Read the model definition and answer for the solid it produces. Units are mm, in the model's axes. A direction names the side the tool comes from. Give positions to 0.01 mm unless a question says otherwise; leave off trailing zeros. Loops run counter-clockwise (first coordinate to the right, second up) from the corner with the lowest first, then second, coordinate; pieces in that order, holes last. Notation, with made-up numbers: (58, 3.5) -> (98, 3.5) arc R22 ccw to (98, 13.5) -> close; hole circle Ø10 at (-26, 79). An arc over 180 degrees is marked (long way). Write each question's results on one line, items separated by ' | '. Start each with the question number.
Item 1: Determine the mould class of faces 5 (the flat face through (50, 47.625, 16)), 6 (the flat face through (101.6, 1, -4)), 7 (the flat face through (76.2, -50, 5)) for opening direction X: +X half, -X half, draft (parallel to the pull), parting line (faces both ways), or undercut.
Item 2: Which of the six approach directions +Z, -Z, +X, -X, +Y, -Y give full straight-line access (tool end or side, diameter ignored) to faces 1 (the flat face through (50, -2, 34.742)), 2 (the flat face through (25.4, -50, 5)), 3 (the flat face through (50, 7, -3.175)), 4 (the flat face through (50.8, -50, 5))?
Item 3: Find the intervals of material crossed by line 1 (Z direction, x = 53.5, y = -26) (3 decimals); line 2 (Z direction, x = 37, y = -50); line 3 (Z direction, x = 72.5, y = -48.5), in increasing order.
Item 4: Section D-D on z = 14.5 is taken. Write down the section's boundary in (x, y) (3 decimals).
Item 5: Section B-B on y = 27 is taken. Write down the section's boundary in (x, z) (3 decimals), and give its area (3 significant figures).
Item 6: Each of these flat-tipped pins is pushed along its axis until it touches: P1, Ø6.5, axis at y = -54, z = 0.5, coming from the -X side; P2, Ø7.5, axis at y = -50.8, z = 0, coming from the -X side; P3, Ø2.5, axis at x = 50.5, z = 36.5, coming from the -Y side. Where does it stop, or does it pass through?
Item 7: Section C-C on x = 68 is taken. Write down the section's boundary in (y, z) (3 decimals), and give its area (3 significant figures).
```python
from build123d import *

# Parameters (mm, degrees)
F1_DEPTH = 101.6
F2_DEPTH = 101.6
F3_DEPTH = 76.2
F4_DEPTH = 50.8
F5_DEPTH = 25.4


with BuildPart() as f1:
    # F0 (on Right) → F1 (new body)
    with BuildSketch(Plane.YZ):
        Polygon((-34.925, -3.175), (-44.45, 6.35), (-44.45, 0), (-44.45, -6.35), (50.8, -6.35), (50.8, 6.35), (50.8, 34.7416847944), (50.8, 37.9166847944), (47.625, 37.9166847944), (-50.8, 37.9166847944), (-50.8, 34.7416847944), (47.625, 34.7416847944), (47.625, 6.35), (47.625, -3.175), align=None)
        with BuildLine():
            Line((-44.45, -6.35), (-44.45, 0))
            ThreePointArc((-44.45, 0), (-46.3098719395, -4.4901280605), (-50.8, -6.35))
            Line((-50.8, -6.35), (-44.45, -6.35))
        make_face()
        with BuildLine():
            Line((-44.45, 0), (-44.45, 6.35))
            Line((-44.45, 6.35), (-50.8, 6.35))
            ThreePointArc((-50.8, 6.35), (-46.3098719395, 4.4901280605), (-44.45, 0))
        make_face()
    extrude(amount=F1_DEPTH)

    # F0 (on Right) → F2 (join)
    with BuildSketch(Plane.YZ):
        with BuildLine():
            ThreePointArc((-44.45, 0), (-46.3098719395, 4.4901280605), (-50.8, 6.35))
            Line((-50.8, 6.35), (-50.8, 4.7625))
            ThreePointArc((-50.8, 4.7625), (-47.4324039546, 3.3675960454), (-46.0375, 0))
            ThreePointArc((-46.0375, 0), (-47.4324039546, -3.3675960454), (-50.8, -4.7625))
            Line((-50.8, -4.7625), (-50.8, -6.35))
            ThreePointArc((-50.8, -6.35), (-46.3098719395, -4.4901280605), (-44.45, 0))
        make_face()
        with BuildLine():
            Line((-50.8, 4.7625), (-50.8, 6.35))
            ThreePointArc((-50.8, 6.35), (-57.15, 0), (-50.8, -6.35))
            Line((-50.8, -6.35), (-50.8, -4.7625))
            ThreePointArc((-50.8, -4.7625), (-55.5625, 0), (-50.8, 4.7625))
        make_face()
    extrude(amount=F2_DEPTH)

    # F0 (on Right) → F3 (cut)
    with BuildSketch(Plane.YZ):
        with BuildLine():
            Line((-50.8, 4.7625), (-50.8, 6.35))
            ThreePointArc((-50.8, 6.35), (-57.15, 0), (-50.8, -6.35))
            Line((-50.8, -6.35), (-50.8, -4.7625))
            ThreePointArc((-50.8, -4.7625), (-55.5625, 0), (-50.8, 4.7625))
        make_face()
        with BuildLine():
            ThreePointArc((-44.45, 0), (-46.3098719395, 4.4901280605), (-50.8, 6.35))
            Line((-50.8, 6.35), (-50.8, 4.7625))
            ThreePointArc((-50.8, 4.7625), (-47.4324039546, 3.3675960454), (-46.0375, 0))
            ThreePointArc((-46.0375, 0), (-47.4324039546, -3.3675960454), (-50.8, -4.7625))
            Line((-50.8, -4.7625), (-50.8, -6.35))
            ThreePointArc((-50.8, -6.35), (-46.3098719395, -4.4901280605), (-44.45, 0))
        make_face()
    extrude(amount=F3_DEPTH, mode=Mode.SUBTRACT)

    # F0 (on Right) → F4 (join)
    with BuildSketch(Plane.YZ):
        with BuildLine():
            Line((-50.8, 4.7625), (-50.8, 6.35))
            ThreePointArc((-50.8, 6.35), (-57.15, 0), (-50.8, -6.35))
            Line((-50.8, -6.35), (-50.8, -4.7625))
            ThreePointArc((-50.8, -4.7625), (-55.5625, 0), (-50.8, 4.7625))
        make_face()
        with BuildLine():
            ThreePointArc((-44.45, 0), (-46.3098719395, 4.4901280605), (-50.8, 6.35))
            Line((-50.8, 6.35), (-50.8, 4.7625))
            ThreePointArc((-50.8, 4.7625), (-47.4324039546, 3.3675960454), (-46.0375, 0))
            ThreePointArc((-46.0375, 0), (-47.4324039546, -3.3675960454), (-50.8, -4.7625))
            Line((-50.8, -4.7625), (-50.8, -6.35))
            ThreePointArc((-50.8, -6.35), (-46.3098719395, -4.4901280605), (-44.45, 0))
        make_face()
    extrude(amount=F4_DEPTH)

    # F0 (on Right) → F5 (cut)
    with BuildSketch(Plane.YZ):
        with BuildLine():
            ThreePointArc((-44.45, 0), (-46.3098719395, 4.4901280605), (-50.8, 6.35))
            Line((-50.8, 6.35), (-50.8, 4.7625))
            ThreePointArc((-50.8, 4.7625), (-47.4324039546, 3.3675960454), (-46.0375, 0))
            ThreePointArc((-46.0375, 0), (-47.4324039546, -3.3675960454), (-50.8, -4.7625))
            Line((-50.8, -4.7625), (-50.8, -6.35))
            ThreePointArc((-50.8, -6.35), (-46.3098719395, -4.4901280605), (-44.45, 0))
        make_face()
        with BuildLine():
            Line((-50.8, 4.7625), (-50.8, 6.35))
            ThreePointArc((-50.8, 6.35), (-57.15, 0), (-50.8, -6.35))
            Line((-50.8, -6.35), (-50.8, -4.7625))
            ThreePointArc((-50.8, -4.7625), (-55.5625, 0), (-50.8, 4.7625))
        make_face()
    extrude(amount=F5_DEPTH, mode=Mode.SUBTRACT)


solid = f1.part
```
Findings:
1) face 5: draft | face 6: +X half | face 7: undercut
2) face 1: +X, -X, -Y | face 2: -X, -Y | face 3: +X, -X | face 4: -Y
3) line 1: -6.35 to -3.175, 34.742 to 37.917 | line 2: -6.35 to -4.69, 4.69 to 6.35, 34.74 to 37.92 | line 3: -6.35 to -5.92, 5.92 to 6.35, 34.74 to 37.92
4) outline: (0, 47.625) -> (101.6, 47.625) -> (101.6, 50.8) -> (0, 50.8) -> close
5) outline: (0, -6.35) -> (101.6, -6.35) -> (101.6, -3.175) -> (0, -3.175) -> close; (0, 34.742) -> (101.6, 34.742) -> (101.6, 37.917) -> (0, 37.917) -> close | area: 645 mm2
6) P1: x = 25.4 | P2: through | P3: y = -50.8
7) outline: (-50.8, -6.35) -> (50.8, -6.35) -> (50.8, 37.917) -> (-50.8, 37.917) -> (-50.8, 34.742) -> (47.625, 34.742) -> (47.625, -3.175) -> (-34.925, -3.175) -> (-44.45, 6.35) -> (-50.8, 6.35) arc R6.35 cw to start | area: 808 mm2
